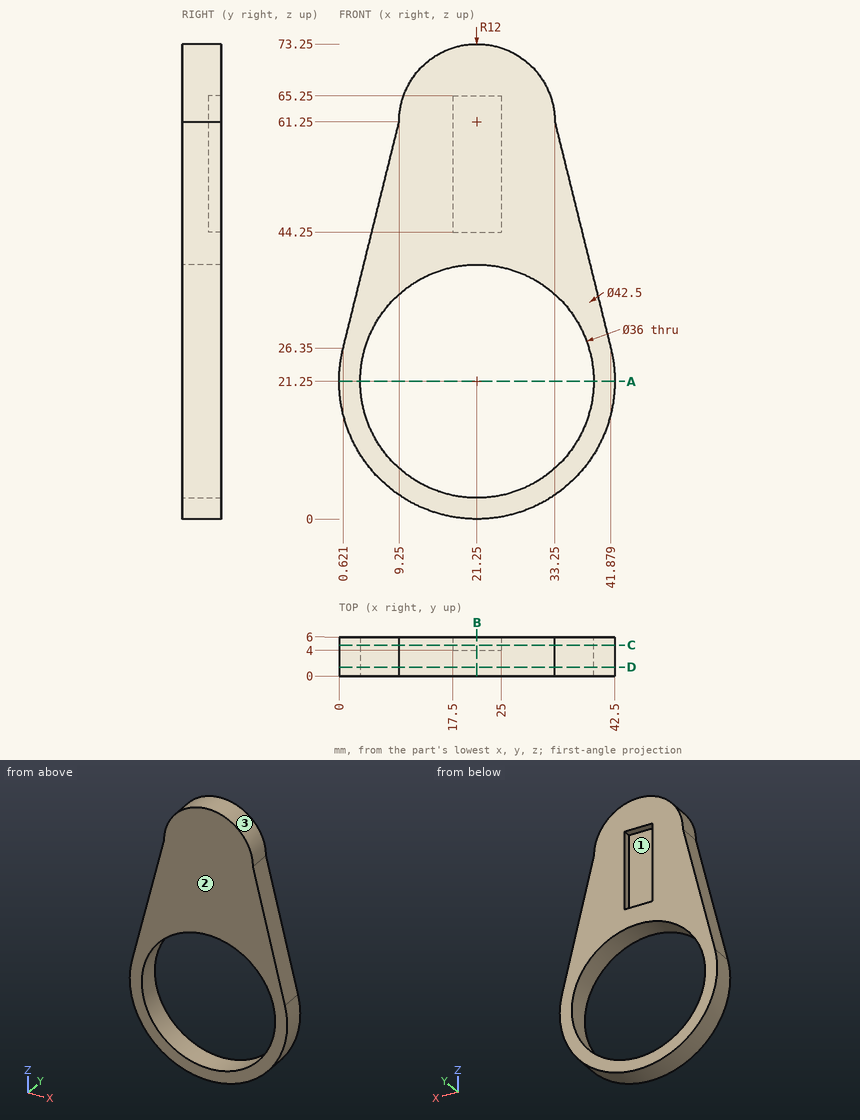
Input: dimensioned drawing with shaded views. Units: mm. Origin: part minimum x, y, z. Coordinates: 2 decimals unless noted, no trailing zeros. Order: outer loops, then holes, each group sorted by start corner. A loop starts at its lowest first (then second) coordinate and runs counter-clockwise, first axis right, second up. Notation, with made-up numbers: M 73.25,56 L 85.25,56 A20 ccw 85.25,89 Z; hole C 85.25,-21.75 d1. An arc over 180 degrees is marked long. Answer as CSV lines item,"result".
Q1. Section D-D on y = 1.35. Return the cut outline in (x, z), and give its area (3 significant figures).
Answers:
outline,"M 0.62,26.35 A21.25 ccw long 41.88,26.35 L 33.25,61.25 A12 ccw 9.25,61.25 Z; hole C 21.25,21.25 d36"
area,"1,270 mm^2"
Q2. Section A-A on z = 21.25. Return the cut outline in (x, y).
Answers:
outline,"M 0,0 L 3.25,0 L 3.25,6 L 0,6 Z; M 39.25,0 L 42.5,0 L 42.5,6 L 39.25,6 Z"
Q3. Line query: probe 1 along X at (y, z) = (4.7, 21.25); probe 2 along Z at (x, y) = (21.25, 3.65); probe 3 along Z at (x, y) = (16, 1.7). Output: solid intervals per line, ascending. Write a range as [from, to].
Answers:
probe 1,"x = [0, 3.25], [39.25, 42.5]"
probe 2,"z = [0, 3.25], [39.25, 73.25]"
probe 3,"z = [0.66, 4.03], [38.47, 72.04]"
Q4. Draft query along X for the marked faces 1, 2 and 3. Return one class per face: pulls with the +X half, pulls with the -X half, needs draft (parallel to the pull), parting line crosses it, or undercut.
Answers:
face 1,"undercut"
face 2,"needs draft"
face 3,"parting line crosses it"
Q5. First-contact query: P1, Ø1.6, axis at x = 21.5, y = 5.5, coming from the -Z side; P2, Ø3, axis at x = 17, y = 5, coming from the +Z side; P3, Ø0.6, axis at y = 4.5, z = 53, coming from the +X side. Flat tips, straight axial feed; report the tip coordinate or a pass-through.
Answers:
P1,"stops at z = 0"
P2,"stops at z = 72.93"
P3,"stops at x = 35.36"
Q6. Section C-C on y = 4.75. Return the cut outline in (x, z).
Answers:
outline,"M 0.62,26.35 A21.25 ccw long 41.88,26.35 L 33.25,61.25 A12 ccw 9.25,61.25 Z; hole C 21.25,21.25 d36; hole M 17.5,44.25 L 25,44.25 L 25,65.25 L 17.5,65.25 Z"
Q7. Section B-B on x = 21.25. Return the cut outline in (y, z).
Answers:
outline,"M 0,0 L 6,0 L 6,3.25 L 0,3.25 Z; M 0,39.25 L 6,39.25 L 6,44.25 L 4,44.25 L 4,65.25 L 6,65.25 L 6,73.25 L 0,73.25 Z"
